```python
from build123d import *

# Parameters (mm, degrees)
SKETCH1_W      = 203.2
SKETCH1_H      = 203.2
EXTRUDE1_DEPTH = 6.35
SKETCH2_R      = 6.2865
EXTRUDE2_DEPTH = 144.824345992
SKETCH3_R      = 1.524
EXTRUDE3_DEPTH = 144.824345992
SKETCH4_W      = 0.79375
SKETCH4_H      = 6.35
EXTRUDE4_DEPTH = 6.35


with BuildPart() as part:
    # Sketch1 → Extrude1 (new body)
    with BuildSketch(Plane.XY):
        Rectangle(SKETCH1_W, SKETCH1_H)
    extrude(amount=EXTRUDE1_DEPTH)

    # Sketch2 → Extrude2 (cut, through all)
    with BuildSketch(Plane.XY.offset(6.35)):
        Circle(SKETCH2_R)
    extrude(amount=-EXTRUDE2_DEPTH, mode=Mode.SUBTRACT)

    # Sketch3 → Extrude3 (cut, through all)
    with BuildSketch(Plane.XY.offset(6.35)):
        with Locations((-47.625, -82.48891971)):
            Circle(SKETCH3_R)
        with Locations((47.625, -82.48891971)):
            Circle(SKETCH3_R)
    extrude(amount=-EXTRUDE3_DEPTH, mode=Mode.SUBTRACT)

    # Sketch4 → Extrude4 (cut)
    with BuildSketch(Plane.XY.offset(6.35)):
        with Locations((0, -98.425)):
            Rectangle(SKETCH4_W, SKETCH4_H)
    extrude(amount=-EXTRUDE4_DEPTH, mode=Mode.SUBTRACT)


solid = part.part
```
The model under review builds one solid part; all positions refer to its coordinate system, in mm. A direction names the side the tool comes from. Give positions to 0.01 mm unless a question says otherwise; leave off trailing zeros. Write each loop counter-clockwise with the first axis right and the second up, starting at its lowest first coordinate (ties: lowest second). Pieces come first, ordered by that corner, then holes. Notation, with made-up numbers: (61, 18.25) - (93, 18.25) arc R36 ccw to (93, 52.25) - close; hole circle Ø8 at (-27.75, 12.5). An arc over 180 degrees is marked (long way). Answer in a Markdown table with one row per item. Add a question column.
1. We need section A-A on y = 0. Write out the cut boundary in (x, z).
2. Draft analysis for pull direction X (two halves, no side actions). For faces 3 (the flat face through (-101.6, -1, 3)), 4 (the flat face through (21, 1, 0)), 5 (the cylindrical face through (-1.363, -6.137, 3.219)), state which applies: +X half, -X half, draft (parallel to the pull), parting line (faces both ways), or undercut.
3. Tool access review of faces 1 (the flat face through (-0.397, -98, 3)), 2 (the flat face through (-52, -101.6, 3)): name each direction out of +Z, -Z, +X, -X, +Y, -Y from which nothing blocks a thin tool from reaching the whole face with its end or side.
4. Wall thickness on line 1 along X through (y, z) = (5.5, 1.5); line 2 along X through (y, z) = (2, 1): over which ranges is each line inside the solid? List them lowest first. Write a range as [from, to].
Ans:
| question | item | result |
|---|---|---|
| 1 | outline | (-101.6, 0) - (-6.29, 0) - (-6.29, 6.35) - (-101.6, 6.35) - close; (6.29, 0) - (101.6, 0) - (101.6, 6.35) - (6.29, 6.35) - close |
| 2 | face 3 | -X half |
| 2 | face 4 | draft |
| 2 | face 5 | undercut |
| 3 | face 1 | +Z, -Z, -Y |
| 3 | face 2 | +Z, -Z, +X, -X, -Y |
| 4 | line 1 | x = [-101.6, -3.04], [3.04, 101.6] |
| 4 | line 2 | x = [-101.6, -5.96], [5.96, 101.6] |
